```python
from build123d import *

# Parameters (mm, degrees)
SKETCH1_W           = 100
SKETCH1_H           = 100
SKETCH1_R           = 2.5
BOSS_EXTRUDE1_DEPTH = 5
CUT_EXTRUDE1_START  = -5
SKETCH6_R           = 4.5
CUT_EXTRUDE1_DEPTH  = 3
SKETCH8_W           = 8
SKETCH8_H           = 35
BOSS_EXTRUDE2_DEPTH = 100
SKETCH9_W           = 100
SKETCH9_H           = 8
BOSS_EXTRUDE3_DEPTH = 210
SKETCH10_W          = 160
SKETCH10_H          = 50
BOSS_EXTRUDE4_DEPTH = 8
SKETCH11_W          = 140
SKETCH11_H          = 30
CUT_EXTRUDE2_DEPTH  = 8
SKETCH13_R          = 1
CUT_EXTRUDE3_DEPTH  = 8
FILLET1_R           = 20
BOSS_EXTRUDE5_DEPTH = 100
FILLET3_R           = 20
SKETCH15_W          = 5
SKETCH15_H          = 100
BOSS_EXTRUDE6_DEPTH = 30


with BuildPart() as part:
    # Sketch1 → Boss-Extrude1 (new body)
    with BuildSketch(Plane(origin=(0, 0, 0), x_dir=(1, 0, 0), z_dir=(0, 1, 0))):
        Rectangle(SKETCH1_W, SKETCH1_H)
        with Locations((-36.95, 36.95)):
            Circle(SKETCH1_R, mode=Mode.SUBTRACT)
        with Locations((36.95, 36.95)):
            Circle(SKETCH1_R, mode=Mode.SUBTRACT)
        with Locations((36.95, -36.95)):
            Circle(SKETCH1_R, mode=Mode.SUBTRACT)
        with Locations((-36.95, -36.95)):
            Circle(SKETCH1_R, mode=Mode.SUBTRACT)
    extrude(amount=BOSS_EXTRUDE1_DEPTH)

    # Sketch6 → Cut-Extrude1 (cut)
    with BuildSketch(Plane.XZ.offset(CUT_EXTRUDE1_START)):
        with Locations((-36.95, 36.95)):
            Circle(SKETCH6_R)
        with Locations((36.95, 36.95)):
            Circle(SKETCH6_R)
        with Locations((36.95, -36.95)):
            Circle(SKETCH6_R)
        with Locations((-36.95, -36.95)):
            Circle(SKETCH6_R)
    extrude(amount=CUT_EXTRUDE1_DEPTH, mode=Mode.SUBTRACT)

    # Sketch8 → Boss-Extrude2 (add, through all)
    with BuildSketch(Plane.ZY.offset(50)):
        with Locations((54, 17.5)):
            Rectangle(SKETCH8_W, SKETCH8_H)
    extrude(amount=-BOSS_EXTRUDE2_DEPTH)

    # Sketch9 → Boss-Extrude3 (add)
    with BuildSketch(Plane.XY.offset(58)):
        with Locations((0, 31)):
            Rectangle(SKETCH9_W, SKETCH9_H)
    extrude(amount=BOSS_EXTRUDE3_DEPTH)

    # Sketch10 → Boss-Extrude4 (add)
    with BuildSketch(Plane(origin=(0, 35, 0), x_dir=(1, 0, 0), z_dir=(0, 1, 0))):
        with Locations((0, -131.95)):
            Rectangle(SKETCH10_W, SKETCH10_H)
    extrude(amount=-BOSS_EXTRUDE4_DEPTH)

    # Sketch11 → Cut-Extrude2 (cut)
    with BuildSketch(Plane(origin=(0, 35, 0), x_dir=(1, 0, 0), z_dir=(0, 1, 0))):
        with Locations((0, -131.95)):
            Rectangle(SKETCH11_W, SKETCH11_H)
    extrude(amount=-CUT_EXTRUDE2_DEPTH, mode=Mode.SUBTRACT)

    # Sketch13 → Cut-Extrude3 (cut)
    with BuildSketch(Plane(origin=(0, 35, 0), x_dir=(1, 0, 0), z_dir=(0, 1, 0))):
        with Locations((-37, -181)):
            Circle(SKETCH13_R)
        with Locations((37, -181)):
            Circle(SKETCH13_R)
        with Locations((37, -255)):
            Circle(SKETCH13_R)
        with Locations((-37, -255)):
            Circle(SKETCH13_R)
    extrude(amount=-CUT_EXTRUDE3_DEPTH, mode=Mode.SUBTRACT)

    # Fillet1
    fillet1_edges = [part.edges().sort_by_distance(p)[0] for p in [
        (50, 31, 156.95),
        (-50, 31, 156.95),
        (50, 31, 106.95),
        (-50, 31, 106.95),
    ]]
    fillet(fillet1_edges, radius=FILLET1_R)

    # Sketch14 → Boss-Extrude5 (add)
    with BuildSketch(Plane.ZY.offset(50)):
        Polygon((58, 0), (58, 27), (68, 27), align=None)
    extrude(amount=-BOSS_EXTRUDE5_DEPTH)

    # Fillet3
    fillet3_edges = [part.edges().sort_by_distance(p)[0] for p in [
        (0, 27, 68),
    ]]
    fillet(fillet3_edges, radius=FILLET3_R)

    # Sketch15 → Boss-Extrude6 (add)
    with BuildSketch(Plane(origin=(0, 5, 0), x_dir=(1, 0, 0), z_dir=(0, 1, 0))):
        with Locations((-47.5, 0)):
            Rectangle(SKETCH15_W, SKETCH15_H)
        with Locations((47.5, 0)):
            Rectangle(SKETCH15_W, SKETCH15_H)
    extrude(amount=BOSS_EXTRUDE6_DEPTH)


solid = part.part
```
Here's how the part is built. I have some questions about the finished solid (model axes, mm). A direction names the side the tool comes from. Coordinates: 2 decimals unless noted, no trailing zeros. Order: outer loops, then holes, each group sorted by start corner. A loop starts at its lowest first (then second) coordinate and runs counter-clockwise, first axis right, second up.
1) Which directions (+Z, -Z, +X, -X, +Y, -Y) give clear straight access to the entire face, cutting with the end or side of a thin tool? Please do faces 1 (the face through (-50, 31, 222)), 2 (the face through (-1, 27, 174)), 3 (the face through (-70, 31, 132)), 4 (the face through (45, 20, 1)), 5 (the face through (39, 2, 35)).
2) Imagine slicing it at A-A on x = -1.5. List the corners of the cut face in (y, z) for me, and give its area (3 significant figures).
3) I need wall thicknesses on line 1 (X direction, y = 33, z = 255); line 2 (Z direction, x = 37, y = 32); line 3 (Z direction, x = -36, y = 1). Which ranges of each line are inside material? Lowest first, please.
4) Will these pins go through, and if not, where does the flat tip stop? pin 1 (9 mm diameter, centred on x = -76.5, y = 30.5, fed in from +Z); pin 2 (4.5 mm diameter, centred on x = -36.95, z = 36.95, fed in from -Y); pin 3 (12 mm diameter, centred on y = 7.5, z = 10, fed in from -X); pin 4 (6.5 mm diameter, centred on x = -75, y = 33, fed in from -Z).
5) Imagine slicing it at D-D on x = -64. List the corners of the cut face in (y, z) for me, and give its area (3 significant figures).
6) We'd pull the mould along Z, two halves only. Please class faces 6 (the face through (-34.531, 3.521, -33.156)), 7 (the face through (50, 31, 222)), 8 (the face through (-34.531, 3.521, 40.744)), 9 (the face through (0.7, 23.32, 70.36)): +Z half, -Z half, draft (parallel to the pull), parting line (faces both ways), or undercut.
7) Imagine slicing it at C-C on z = 194. List the corners of the cut face in (x, y) for me, and give its area (3 significant figures).
8) Imagine slicing it at B-B on y = 8.5. List the corners of the cut face in (x, z) for me.
Response values:
1. face 1: +Z, -X, +Y, -Y
1. face 2: +Z, +X, -X, -Y
1. face 3: +Y, -Y
1. face 4: -Z, +Y
1. face 5: +Y
2. outline: (0, -50) - (5, -50) - (5, 50) - (35, 50) - (35, 116.95) - (27, 116.95) - (27, 81.92) arc R20 cw to (13.95, 63.17) - (0, 58) - close; (27, 146.95) - (35, 146.95) - (35, 268) - (27, 268) - close
2. area: 2,390 mm2
3. line 1: x = -50 to -38, -36 to 36, 38 to 50
3. line 2: z = 50 to 116.95, 146.95 to 180, 182 to 254, 256 to 268
3. line 3: z = -50 to -39.26, -34.64 to 34.64, 39.26 to 58.37
4. pin 1: stops at z = 156.95
4. pin 2: passes through
4. pin 3: stops at x = -50
4. pin 4: stops at z = 106.95
5. outline: (27, 106.03) - (35, 106.03) - (35, 116.95) - (27, 116.95) - close; (27, 146.95) - (35, 146.95) - (35, 157.87) - (27, 157.87) - close
5. area: 175 mm2
6. face 6: undercut
6. face 7: draft
6. face 8: undercut
6. face 9: +Z half
7. outline: (-50, 27) - (50, 27) - (50, 35) - (-50, 35) - close
7. area: 800 mm2
8. outline: (-50, -50) - (-45, -50) - (-45, 50) - (45, 50) - (45, -50) - (50, -50) - (50, 61.15) - (-50, 61.15) - close
